Can you work these out from the drawing? Everything is in mm from the part's minimum corner. A direction names the side the tool comes from. Give positions to 0.01 mm unless a question says otherwise; leave off trailing zeros. Loops run counter-clockwise (first coordinate to the right, second up) from the corner with the lowest first, then second, coordinate; pieces in that order, holes last. Notation, with made-up numbers: (35, -33.75) -> (85, -33.75) arc R17 cw to (85, -24.75) -> close; hole circle Ø2 at (-8.75, 59). An arc over 180 degrees is marked (long way). Return JSON: item names as keys, results as strings. Group by question number.
Q1. I need wall thicknesses on line 1 along Y through (x, z) = (2.25, 0.3); line 2 along X through (y, z) = (17, 2.8); line 3 along Z through (x, y) = (1.55, 13). Which ranges of each line are inside material? Lowest first, please. Write a range as [from, to].
Q2. Suppose I cut it at C-C, the plane y = 3. Please give me the cut outline in (x, z).
Q3. Will these pins go through, and if not, where does the flat tip stop? pin 1 (2 mm diameter, centred on y = 13.5, z = 3.5, fed in from -X); pin 2 (1.5 mm diameter, centred on x = 1, y = 15, fed in from +Z); pin 3 (3 mm diameter, centred on y = 11.5, z = 2, fed in from +X).
Q4. Suppose I cut it at A-A, the plane x = 2.9. Please give me the cut outline in (y, z).
Q5. Which directions (+Z, -Z, +X, -X, +Y, -Y) give clear straight access to the entire face, cutting with the end or side of a thin tool? Please do the marked faces 1 and 2.
Q6. Thinking about a two-plate mould opening in X: for the marked faces 3 and 4, which applies, pulls with the +X half, pulls with the -X half, needs draft (parallel to the pull), parting line crosses it, or undercut?
Q7. Suppose I cut it at B-B, the plane z = 2.9. Please give me the cut outline in (x, y).
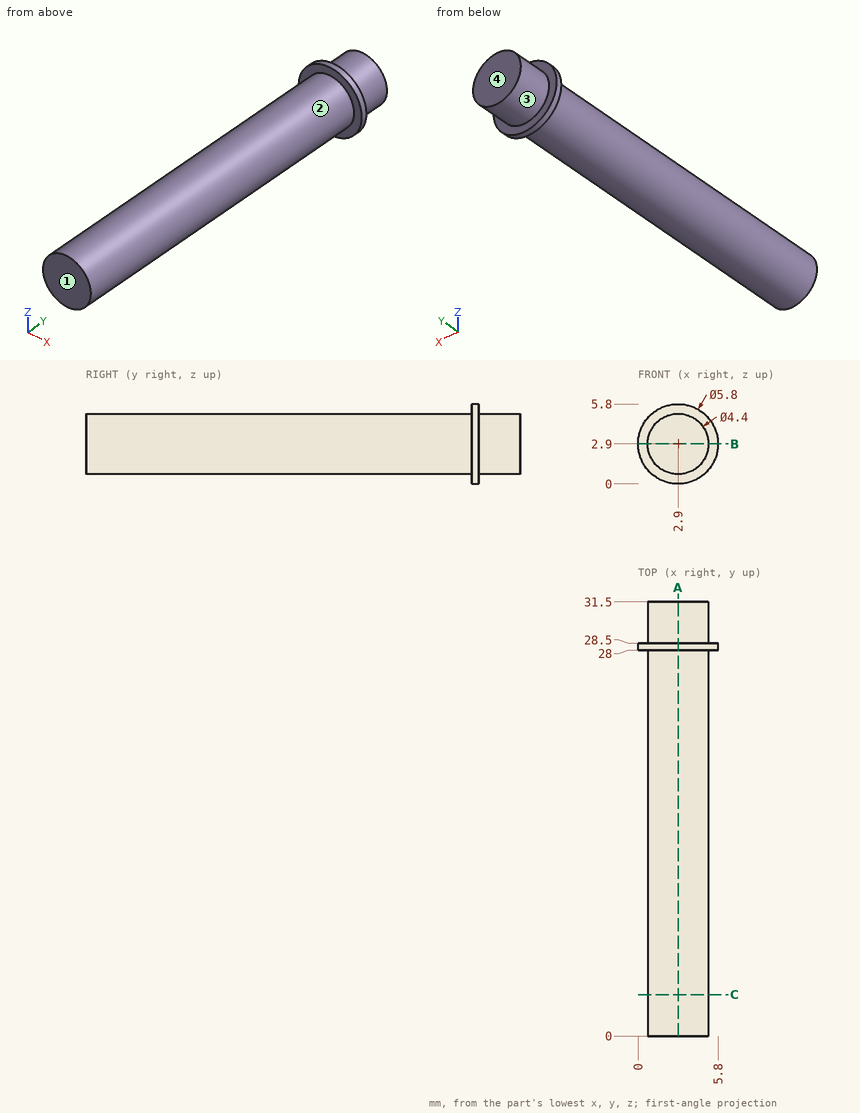
Ans:
{
 "1": {"line 1": "y = [28, 28.5]", "line 2": "x = [0.7, 5.1]", "line 3": "z = [1.16, 4.64]"},
 "2": {"outline": "circle Ø4.4 at (2.9, 2.9)"},
 "3": {"pin 1": "stops at x = 0.7", "pin 2": "stops at z = 4.78", "pin 3": "stops at x = 5.1"},
 "4": {"outline": "(0, 0.7) -> (28, 0.7) -> (28, 0) -> (28.5, 0) -> (28.5, 0.7) -> (31.5, 0.7) -> (31.5, 5.1) -> (28.5, 5.1) -> (28.5, 5.8) -> (28, 5.8) -> (28, 5.1) -> (0, 5.1) -> close"},
 "5": {"face 1": "+Z, -Z, +X, -X, -Y", "face 2": "-Y"},
 "6": {"face 3": "parting line crosses it", "face 4": "needs draft"},
 "7": {"outline": "(0, 28) -> (0.7, 28) -> (0.7, 0) -> (5.1, 0) -> (5.1, 28) -> (5.8, 28) -> (5.8, 28.5) -> (5.1, 28.5) -> (5.1, 31.5) -> (0.7, 31.5) -> (0.7, 28.5) -> (0, 28.5) -> close"}
}
